CAD build for the part. Positions are in the model's coordinates, mm. Face numbers are marked on the shaded views. A direction names the side the tool comes from. Coordinates: 2 decimals unless noted, no trailing zeros. Write each loop counter-clockwise with the first axis right and the second up, starting at its lowest first coordinate (ties: lowest second). Pieces come first, ordered by that corner, then holes. Notation, with made-up numbers: (34, -4.5) - (71, -4.5) arc R18 ccw to (71, 30.5) - close; hole circle Ø6 at (51.5, 50.5). An arc over 180 degrees is marked (long way). Answer in a Markdown table with one row per item. Add a question column.
Q1. Two-plate mould, pull along X, no slides. Class the marked faces 3, 4, 5 and 6: +X half, -X half, draft (parallel to the pull), parting line (faces both ways), or undercut.
Q2. Band-saw the part on C-C (z = -4.5). List the corners of the cut face in (x, y), and give its area (3 significant figures).
Q3. Band-saw the part on B-B (x = -15). List the corners of the cut face in (y, z).
Q4. Drill centre lines: line 1 along Y through (x, z) = (-15, -33.05); line 2 along Y through (x, z) = (-15, -40.75); line 3 along Z through (x, y) = (-28.25, 23). Where is each one in solid material? Low to high. Write a range as from..to.
Q5. Band-saw the part on D-D (y = 16). List the corners of the cut face in (x, z).
Q6. Pin check, flat tips, straight feed: pin 1 (9 mm diameter, centred on x = -13.5, y = 16, fed in from -Z); pin 2 (7.5 mm diameter, centred on x = -10.5, z = -16.5, fed in from +Y); pin 3 (10 mm diameter, centred on y = 24, z = 0.5, fed in from -X); pin 4 (3 mm diameter, centred on x = -14, z = -3, fed in from -Y). Stop position of each tip, or through.
Q7. 3-axis set-ups, long thin cutter, end or side, ignore diameter. For the marked faces 1 and 2: which of +Z, -Z, +X, -X, +Y, -Y reach the whole face in a straight line?
Q8. Band-saw the part on A-A (y = 6). List the corners of the cut face in (x, z).
```python
from build123d import *

# Parameters (mm, degrees)
SALIENTE_EXTRUIR1_DEPTH = 6
CROQUIS3_R              = 4
CORTAR_EXTRUIR1_DEPTH   = 47.013232879
CROQUIS4_R              = 11
CORTAR_EXTRUIR2_DEPTH   = 8.5
CROQUIS5_R              = 10
CORTAR_EXTRUIR3_DEPTH   = 8.5
CROQUIS6_W              = 30
CROQUIS6_H              = 3.5
SALIENTE_EXTRUIR2_DEPTH = 25


with BuildPart() as part:
    # Croquis2 → Saliente-Extruir1 (new, symmetric)
    with BuildSketch(Plane.XY):
        with BuildLine():
            Line((0, 0), (-30, 0))
            Line((-30, 0), (-30, 17.76))
            ThreePointArc((-30, 17.76), (-15, 32.76), (0, 17.76))
            Line((0, 17.76), (0, 0))
        make_face()
    saliente_extruir1 = extrude(amount=SALIENTE_EXTRUIR1_DEPTH, both=True)

    # Croquis3 → Cortar-Extruir1 (cut, through all)
    with BuildSketch(Plane.XY.offset(6)):
        with Locations((-15, 17.76)):
            Circle(CROQUIS3_R)
    extrude(amount=-CORTAR_EXTRUIR1_DEPTH, mode=Mode.SUBTRACT)

    # Croquis4 → Cortar-Extruir2 (cut)
    with BuildSketch(Plane.XY.offset(6)):
        with Locations((-15, 17.76)):
            Circle(CROQUIS4_R)
    cortar_extruir2 = extrude(amount=-CORTAR_EXTRUIR2_DEPTH, mode=Mode.SUBTRACT)

    # Croquis5 → Cortar-Extruir3 (cut)
    with BuildSketch(Plane.XY.offset(-2.5)):
        with Locations((-15, 17.76)):
            Circle(CROQUIS5_R)
    cortar_extruir3 = extrude(amount=-CORTAR_EXTRUIR3_DEPTH, mode=Mode.SUBTRACT)

    # Croquis6 → Saliente-Extruir2 (add)
    with BuildSketch(Plane(origin=(0, 0, -6), x_dir=(-1, 0, 0), z_dir=(0, 0, -1))):
        with Locations((15, 1.75)):
            Rectangle(CROQUIS6_W, CROQUIS6_H)
    extrude(amount=SALIENTE_EXTRUIR2_DEPTH)

    # Simetría1: Saliente-Extruir1, Cortar-Extruir2, Cortar-Extruir3 across plane
    add(saliente_extruir1.mirror(Plane(origin=(0, 0, -18.5), x_dir=(1, 0, 0), z_dir=(0, 0, -1))))
    add(cortar_extruir2.mirror(Plane(origin=(0, 0, -18.5), x_dir=(1, 0, 0), z_dir=(0, 0, -1))), mode=Mode.SUBTRACT)
    add(cortar_extruir3.mirror(Plane(origin=(0, 0, -18.5), x_dir=(1, 0, 0), z_dir=(0, 0, -1))), mode=Mode.SUBTRACT)


solid = part.part
```
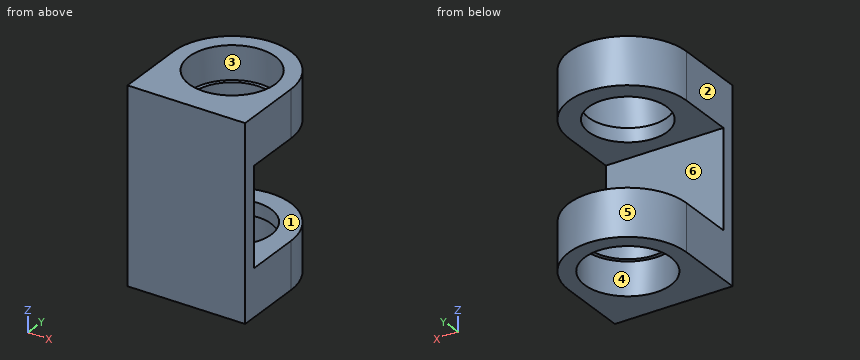
Checked values:
| question | item | result |
|---|---|---|
| 1 | face 3 | undercut |
| 1 | face 4 | undercut |
| 1 | face 5 | parting line |
| 1 | face 6 | draft |
| 2 | outline | (-30, 0) - (0, 0) - (0, 17.76) arc R15 ccw to (-30, 17.76) - close; hole circle Ø20 at (-15, 17.76) |
| 2 | area | 572 mm² |
| 3 | outline | (0, -43) - (6.76, -43) - (6.76, -34.5) - (7.76, -34.5) - (7.76, -31) - (3.5, -31) - (3.5, -6) - (7.76, -6) - (7.76, -2.5) - (6.76, -2.5) - (6.76, 6) - (0, 6) - close; (27.76, -34.5) - (28.76, -34.5) - (28.76, -43) - (32.76, -43) - (32.76, -31) - (27.76, -31) - close; (27.76, -6) - (32.76, -6) - (32.76, 6) - (28.76, 6) - (28.76, -2.5) - (27.76, -2.5) - close |
| 4 | line 1 | y = 0..7.76, 27.76..32.76 |
| 4 | line 2 | y = 0..6.76, 28.76..32.76 |
| 4 | line 3 | z = -43..-31, -6..6 |
| 5 | outline | (-30, -43) - (-25.86, -43) - (-25.86, -34.5) - (-24.84, -34.5) - (-24.84, -31) - (-30, -31) - close; (-30, -6) - (-24.84, -6) - (-24.84, -2.5) - (-25.86, -2.5) - (-25.86, 6) - (-30, 6) - close; (-5.16, -34.5) - (-4.14, -34.5) - (-4.14, -43) - (0, -43) - (0, -31) - (-5.16, -31) - close; (-5.16, -6) - (0, -6) - (0, 6) - (-4.14, 6) - (-4.14, -2.5) - (-5.16, -2.5) - close |
| 6 | pin 1 | passes through |
| 6 | pin 2 | stops at y = 3.5 |
| 6 | pin 3 | stops at x = -29.95 |
| 6 | pin 4 | stops at y = 0 |
| 7 | face 1 | +X, -X, +Y |
| 7 | face 2 | +Z, -Z, -X, +Y, -Y |
| 8 | outline | (-30, -43) - (0, -43) - (0, -31) - (-30, -31) - close; (-30, -6) - (0, -6) - (0, 6) - (-30, 6) - close |
